Check sheet for the modelled part. Datum: model origin and axes. Units: mm. Coordinates: 2 decimals unless noted, no trailing zeros. Write each loop counter-clockwise with the first axis right and the second up, starting at its lowest first coordinate (ties: lowest second). Pieces come first, ordered by that corner, then holes. Notation, with made-up numbers: M 69.25,20.5 L 73.25,20.5 A11 cw 73.25,39.5 Z; hole C -15.75,54.25 d6. An arc over 180 degrees is marked long. Answer as CSV lines item,"result".
from build123d import *

# Parameters (mm, degrees)
SKETCH_1_W          = 220
SKETCH_1_H          = 54
SKETCH_1_R          = 2.1
EXTRUDE_1_DEPTH     = 2.5
CHAMFER_1_SIZE      = 4
CHAMFER_2_SIZE      = 2
SKETCH_3_R          = 2
CUT_EXTRUDE_1_DEPTH = 114.375482358
SKETCH_4_R          = 30
CUT_EXTRUDE_2_DEPTH = 114.375482358
FILLET_1_R          = 10
EXTRUDE_2_DEPTH     = 5
FILLET_2_R          = 1


with BuildPart() as part:
    # 草图1 → 凸台-拉伸1 (new, symmetric)
    with BuildSketch(Plane.XY):
        Rectangle(SKETCH_1_W, SKETCH_1_H)
        with Locations((-100, 17)):
            Circle(SKETCH_1_R, mode=Mode.SUBTRACT)
        with Locations((-100, -17)):
            Circle(SKETCH_1_R, mode=Mode.SUBTRACT)
        with Locations((100, 17)):
            Circle(SKETCH_1_R, mode=Mode.SUBTRACT)
        with Locations((100, -17)):
            Circle(SKETCH_1_R, mode=Mode.SUBTRACT)
        with Locations((-12.25, 22)):
            Circle(SKETCH_1_R, mode=Mode.SUBTRACT)
        with Locations((12.25, 22)):
            Circle(SKETCH_1_R, mode=Mode.SUBTRACT)
    extrude(amount=EXTRUDE_1_DEPTH, both=True)

    # 倒角1
    chamfer_1_edges = [part.edges().sort_by_distance(p)[0] for p in [
        (-110, 27, 0),
        (110, 27, 0),
        (110, -27, 0),
        (-110, -27, 0),
    ]]
    chamfer(chamfer_1_edges, length=CHAMFER_1_SIZE)

    # 倒角2
    chamfer_2_edges = [part.edges().sort_by_distance(p)[0] for p in [
        (-102.1, 17, 2.5),
        (-102.1, -17, 2.5),
        (97.9, 17, 2.5),
        (97.9, -17, 2.5),
        (-14.35, 22, -2.5),
        (10.15, 22, -2.5),
    ]]
    chamfer(chamfer_2_edges, length=CHAMFER_2_SIZE)

    # 草图3 → 切除-拉伸1 (cut, through all)
    with BuildSketch(Plane.XY.offset(2.5)):
        with Locations((50.753537587, -17)):
            Circle(SKETCH_3_R)
        with Locations((41.643265044, 17)):
            Circle(SKETCH_3_R)
        with Locations((30.753537587, -17)):
            Circle(SKETCH_3_R)
        with Locations(Location((-41.643265044, 17, 0), (0, 0, 180))):
            Circle(SKETCH_3_R)
        with Locations(Location((-50.753537587, -17, 0), (0, 0, 180))):
            Circle(SKETCH_3_R)
        with Locations(Location((-30.753537587, -17, 0), (0, 0, 180))):
            Circle(SKETCH_3_R)
    extrude(amount=-CUT_EXTRUDE_1_DEPTH, mode=Mode.SUBTRACT)

    # 草图4 → 切除-拉伸2 (cut, through all)
    with BuildSketch(Plane.XY.offset(2.5)):
        with Locations((0, -46)):
            Circle(SKETCH_4_R)
    extrude(amount=-CUT_EXTRUDE_2_DEPTH, mode=Mode.SUBTRACT)

    # 圆角1
    fillet_1_edges = [part.edges().sort_by_distance(p)[0] for p in [
        (23.216373532, -27, 0),
        (-23.216373532, -27, 0),
    ]]
    fillet(fillet_1_edges, radius=FILLET_1_R)

    # 草图5 → 凸台-拉伸2 (add)
    with BuildSketch(Plane(origin=(0, 0, -2.5), x_dir=(-1, 0, 0), z_dir=(0, 0, -1))):
        Polygon((-21.5, 42), (21.5, 42), (30.160254038, 27), (-30.160254038, 27), align=None)
    extrude(amount=-EXTRUDE_2_DEPTH)

    # 圆角2
    fillet_2_edges = [part.edges().sort_by_distance(p)[0] for p in [
        (-30.160254038, 27, 0),
        (-21.5, 42, 0),
        (21.5, 42, 0),
        (30.160254038, 27, 0),
    ]]
    fillet(fillet_2_edges, radius=FILLET_2_R)


solid = part.part
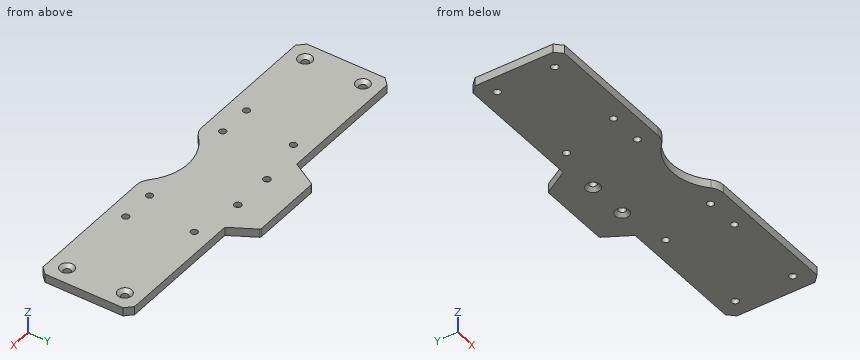
1) Section check B-B, the plane x = -12.25. Record the boundary of the cut face in (y, z).
Answer key:
outline,"M -18.62,-2.5 L 17.9,-2.5 L 19.9,-0.5 L 19.9,2.5 L -18.62,2.5 Z; M 24.1,-0.5 L 26.1,-2.5 L 42,-2.5 L 42,2.5 L 24.1,2.5 Z"
2) Thickness scan on line 1 along Y through (x, z) = (-100, -0.7); line 2 along X through (y, z) = (22.5, 0.85); line 3 along Y through (x, z) = (0, 1.85). Record the ranges inside material, lowest first.
Answer key:
line 1,"y = -27 to -19.1, -14.9 to 14.9, 19.1 to 27"
line 2,"x = -110 to -14.29, -10.21 to 10.21, 14.29 to 110"
line 3,"y = -16 to 42"
3) Section check C-C, the plane x = -81. Record the boundary of the cut face in (y, z), plus the area to 3 significant figures.
Answer key:
outline,"M -27,-2.5 L 27,-2.5 L 27,2.5 L -27,2.5 Z"
area,"270 mm2"
4) Section check A-A, the plane x = 100. Record the boundary of the cut face in (y, z), plus the area to 3 significant figures.
Answer key:
outline,"M -27,-2.5 L -19.1,-2.5 L -19.1,0.5 L -21.1,2.5 L -27,2.5 Z; M -14.9,-2.5 L 14.9,-2.5 L 14.9,0.5 L 12.9,2.5 L -12.9,2.5 L -14.9,0.5 Z; M 19.1,-2.5 L 27,-2.5 L 27,2.5 L 21.1,2.5 L 19.1,0.5 Z"
area,"220 mm2"
5) Depth check by flat-ended pin: P1, Ø5.5, axis at x = -100, y = 17, coming from the +Z side; P2, Ø4, axis at x = 100, y = -17, coming from the +Z side; P3, Ø1, axis at y = 33, z = 1, coming from the +X side; P4, Ø5.5, axis at x = 12.25, y = 22, coming from the -Z side. Enter the tip coordinate at first touch or a pass-through.
Answer key:
P1,"stops at z = 1.15"
P2,"passes through"
P3,"stops at x = 26.98"
P4,"stops at z = -1.15"
